```python
from build123d import *

# Parameters (mm, degrees)
BOSS_EXTRUDE1_DEPTH        = 12.7
HOLE1_D                    = 3.175
HOLE1_DEPTH                = 31.75
HOLE1_CSINK_D              = 10.16
HOLE1_CSINK_ANGLE          = 82
HOLE1_TIP                  = 0.953866233
HOLE2_D                    = 3.175
HOLE2_DEPTH                = 31.75
HOLE2_CSINK_D              = 10.16
HOLE2_CSINK_ANGLE          = 82
HOLE2_TIP                  = 0.953866233
F_1_1_DIAMETER_HOLE1_D     = 25.4
F_1_1_DIAMETER_HOLE1_DEPTH = 12.7
F_6_CLEARANCE_HOLE1_D      = 4.3053
F_6_CLEARANCE_HOLE1_DEPTH  = 12.7


with BuildPart() as part:
    # Sketch1 → Boss-Extrude1 (new body)
    with BuildSketch(Plane.XY):
        Polygon((341.304465963, 12.7), (244.004465963, 12.7), (244.004465963, -144.6), (124.004465969, -144.6), (124.004465969, -427.342121692), (341.304465963, -427.342121692), align=None)
    boss_extrude1 = extrude(amount=BOSS_EXTRUDE1_DEPTH)

    # Mirror1: Boss-Extrude1 across plane
    add(boss_extrude1.mirror(Plane(origin=(124.004465969, -144.6, 12.7), x_dir=(0, 0, 1), z_dir=(1, 0, 0))))

    # Hole1
    with Locations(Plane(origin=(124.004465969, 10.424290059, 12.7), x_dir=(-1, 0, 0), z_dir=(0, 0, 1))):
        with Locations((-207.774999994, 333.02141023), (-207.774999994, 225.48903684), (-207.774999994, 137.424290059), (-172.166666661, 4.074290059), (-146.083333327, 4.074290059), (-94.599999994, 161.374290059), (94.599999994, 161.374290059), (146.083333327, 4.074290059), (172.166666661, 4.074290059), (207.774999994, 137.424290059), (207.774999994, 225.48903684), (207.774999994, 333.02141023), (166.795833328, 301.970350905), (40.979166666, 301.970350905), (-40.979166666, 301.970350905), (-166.795833328, 301.970350905), (0, 193.124290059), (0, 301.970350905), (0, 412.366411751), (-126.349999994, 106.824290059), (-126.349999994, 58.624290059), (126.349999994, 58.624290059), (126.349999994, 106.824290059)):
            CounterSinkHole(HOLE1_D / 2, HOLE1_CSINK_D / 2, depth=HOLE1_DEPTH, counter_sink_angle=HOLE1_CSINK_ANGLE)
            with Locations((0, 0, -(HOLE1_DEPTH + HOLE1_TIP / 2))):  # 118° drill point
                Cone(0, HOLE1_D / 2, HOLE1_TIP, mode=Mode.SUBTRACT)

    # Hole2
    with Locations(Plane(origin=(124.004465969, 10.424290059, 0), x_dir=(1, 0, 0), z_dir=(0, 0, -1))):
        with Locations((-155.949999994, 107.734820482), (155.949999994, 107.734820482), (155.949999994, 327.755881328), (174.999999994, 85.732714397), (174.999999994, 349.757987412), (-174.999999994, 349.757987412), (-174.999999994, 85.732714397), (-155.949999994, 327.755881328)):
            CounterSinkHole(HOLE2_D / 2, HOLE2_CSINK_D / 2, depth=HOLE2_DEPTH, counter_sink_angle=HOLE2_CSINK_ANGLE)
            with Locations((0, 0, -(HOLE2_DEPTH + HOLE2_TIP / 2))):  # 118° drill point
                Cone(0, HOLE2_D / 2, HOLE2_TIP, mode=Mode.SUBTRACT)

    # 1 (1) Diameter Hole1
    with Locations(Plane(origin=(0, 0, 0), x_dir=(-1, 0, 0), z_dir=(0, 0, -1))):
        with Locations((-251.379465963, -231.121997256)):
            Hole(F_1_1_DIAMETER_HOLE1_D / 2, depth=F_1_1_DIAMETER_HOLE1_DEPTH)

    # #6 Clearance Hole1
    with Locations(Plane(origin=(0, 0, 0), x_dir=(-1, 0, 0), z_dir=(0, 0, -1))):
        with Locations((-215.152465963, -254.856060846), (-170.702465963, -210.406060846)):
            Hole(F_6_CLEARANCE_HOLE1_D / 2, depth=F_6_CLEARANCE_HOLE1_DEPTH)


solid = part.part
```
Design review of the part built by this model. Coordinates are the model's own, in mm. Coordinates: 2 decimals unless noted, no trailing zeros. Order: outer loops, then holes, each group sorted by start corner. A loop starts at its lowest first (then second) coordinate and runs counter-clockwise, first axis right, second up. Notation, with made-up numbers: M 83.5,-14 L 139.5,-14 A26 cw 139.5,24 Z; hole C -23.5,35 d11. An arc over 180 degrees is marked long. Answer as a JSON object with one key per item and string values. Group by question number.
1) Add section A-A, the plane x = 231. Write out the cut boundary in (y, z), then the cut area to 3 significant figures.
2) Add section B-B, the plane z = 6.25. Count the separate pieces of the cut face and the enclosed holes in it, then the cut area to 3 significant figures.
3) Mouldability with a two-part tool opening along X and no side actions: class faces 1 (the flat face through (-93.296, -210, 6)), 2 (the flat face through (293, 12.7, 6)), 3 (the conical face through (123.62, -289.83, 8.88)) as pulls with the +X half, pulls with the -X half, needs draft (parallel to the pull), parting line crosses it, or undercut.
4) For pin 1 (2.5 mm diameter, centred on x = 218.6, y = -150.95, fed in from -Z); pin 2 (1 mm diameter, centred on x = 11.5, z = 3.5, fed in from +Y); pin 3 (3.5 mm diameter, centred on x = 296.17, y = 6.35, fed in from +Z); pin 4 (5 mm diameter, centred on x = 124, y = -401.94, fed in from +Z), all flat-tipped, find the tip position at first contact; note any pin that passes through.
5) Wall thickness on L1, parallel to Y at x = -22.5, z = 5.5; L2, parallel to X at y = -66.5, z = 2.75; L3, parallel to Y at x = 279, z = 11.25: over which ranges is each line inside the solid? List them lowest first.
Computed values:
{
 "1": {"outline": "M -427.34,0 L -144.6,0 L -144.6,12.7 L -427.34,12.7 Z", "area": "3,590 mm^2"},
 "2": {"separate pieces": "1", "enclosed holes": "34", "area": "153,000 mm^2"},
 "3": {"face 1": "pulls with the -X half", "face 2": "needs draft", "face 3": "undercut"},
 "4": {"pin 1": "passes through", "pin 2": "stops at y = -144.6", "pin 3": "stops at z = 8.87", "pin 4": "stops at z = 9.74"},
 "5": {"L1": "y = -427.34 to 4.82, 7.88 to 12.7", "L2": "x = -93.3 to 4, 244 to 341.3", "L3": "y = -427.34 to -318.6, -316.06 to -98.58, -96.04 to 12.7"}
}
